Check sheet for the modelled part. Datum: model origin and axes. Units: mm. Face numbers are marked on the shaded views. A direction names the side the tool comes from. Coordinates: 2 decimals unless noted, no trailing zeros. Write each loop counter-clockwise with the first axis right and the second up, starting at its lowest first coordinate (ties: lowest second). Pieces come first, ordered by that corner, then holes. Notation, with made-up numbers: (77.25, 5) -> (127.25, 5) arc R21 cw to (127.25, 24) -> close; hole circle Ø5 at (10, 52.5). An arc over 180 degrees is marked (long way). One line per item, written item: value. Start each with the question number.
1) Sectioned sample at B-B on z = -14.25. Enter the section's corners in (x, y).
2) Sectioned sample at C-C on y = -8.25. Enter the section's corners in (x, z) (3 decimals), plus the area to 3 significant figures.
3) Sectioned sample at D-D on x = 11. Enter the section's corners in (y, z).
4) Set-up check for the marked faces 4, 5, 6, 7 and 8: record each of +Z, -Z, +X, -X, +Y, -Y from which the full face is reachable in a straight line by a thin tool's end or side.
5) Sectioned sample at A-A on x = 28. Enter the section's corners in (y, z).
6) Scan lines: line 1 along Y through (x, z) = (6, -6); line 2 along Z through (x, y) = (20, -3); line 3 along X through (y, z) = (-11.5, -10.75). Record each from-to range of solid material in increasing order. Write a range as [from, to].
7) Gauge pin test, flat ends, axial feed: P1, Ø4, axis at x = 27, y = -6, coming from the -Z side; P2, Ø11, axis at x = 25, z = 4, coming from the -Y side; P3, Ø1, axis at y = -15, z = 2, coming from the +X side; P4, Ø7.5, axis at x = -21.09, z = 1.52, coming from the +Y side. Record the tip position at first contact, or that the pin passes through.
8) Draft check along X on the marked faces 1, 2 and 3. Enter one of: +X half, -X half, draft (parallel to the pull), parting line (faces both ways), or undercut.
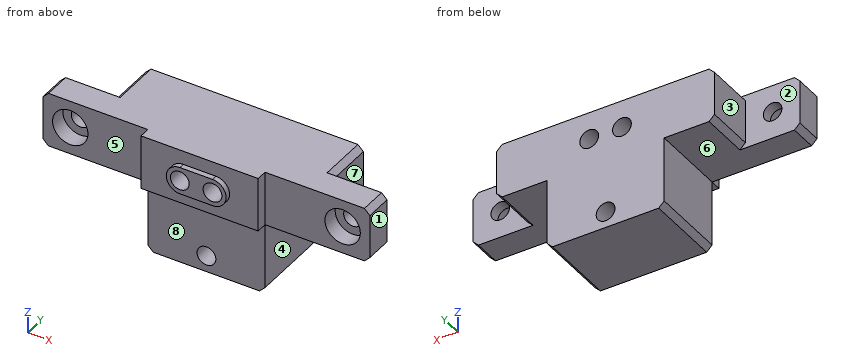
```python
from build123d import *

# Parameters (mm, degrees)
F1_DEPTH  = 16
F2_W      = 21.5
F2_H      = 13
F2_W_2    = 19.25
F2_H_2    = 10
F3_DEPTH  = 2
F4_R      = 3.25
F5_DEPTH  = 3
F6_R      = 1.7
F7_R      = 1.7
F8_DEPTH  = 25
F9_W      = 10
F9_H      = 10
F9_R      = 1.7
F10_DEPTH = 9
F13_DEPTH = 17
F11_R     = 1.725
F14_DEPTH = 15
F15_R     = 1.725
F16_DEPTH = 25
F17_SIZE  = 1


with BuildPart() as f1:
    # F0 (on Front) → F1 (new body)
    with BuildSketch(Plane.XZ):
        Polygon((33.9145704359, 6.5189368035), (-26.0854295641, 6.5189368035), (-26.0854295641, -3.4810631965), (-6.8354295641, -3.4810631965), (-6.8354295641, -16.4810631965), (14.6645704359, -16.4810631965), (14.6645704359, -3.4810631965), (33.9145704359, -3.4810631965), align=None)
    extrude(amount=F1_DEPTH)

    # F2 (on face) → F3 (cut)
    with BuildSketch(Plane.XZ.offset(16)):
        with Locations((3.9145704359, -9.9810631965)):
            Rectangle(F2_W, F2_H)
        with Locations((-16.4604295641, 1.5189368035)):
            Rectangle(F2_W_2, F2_H_2)
        with Locations((24.2895704359, 1.5189368035)):
            Rectangle(F2_W_2, F2_H_2)
    extrude(amount=-F3_DEPTH, mode=Mode.SUBTRACT)

    # F4 (on face) → F5 (cut)
    with BuildSketch(Plane.XZ.offset(14)):
        with Locations((-21.0854295641, 1.5189368035)):
            Circle(F4_R)
        with Locations((28.9145704359, 1.5189368035)):
            Circle(F4_R)
    extrude(amount=-F5_DEPTH, mode=Mode.SUBTRACT)

    # F6 (on face) + F7 (on face) → F8 (cut)
    with BuildSketch(Plane.XZ.offset(11)):
        with Locations((-21.0854295641, 1.5189368035)):
            Circle(F6_R)
    with BuildSketch(Plane.XZ.offset(11)):
        with Locations((28.9145704359, 1.5189368035)):
            Circle(F7_R)
    extrude(amount=-F8_DEPTH, mode=Mode.SUBTRACT)

    # F9 (on face) → F10 (cut)
    with BuildSketch(Plane(origin=(0, 0, 0), x_dir=(-1, 0, 0), z_dir=(0, 1, 0))):
        with Locations((21.0854295641, 1.5189368035)):
            Rectangle(F9_W, F9_H)
        with Locations((21.0854295641, 1.5189368035)):
            Circle(F9_R, mode=Mode.SUBTRACT)
        with Locations((-28.9145704359, 1.5189368035)):
            Rectangle(F9_W, F9_H)
        with Locations((-28.9145704359, 1.5189368035)):
            Circle(F9_R, mode=Mode.SUBTRACT)
    extrude(amount=-F10_DEPTH, mode=Mode.SUBTRACT)

    # F12 (on Front) → F13 (join)
    with BuildSketch(Plane.XZ):
        with BuildLine():
            Line((0.9346461738, -0.9810631965), (6.9134989753, -0.9810631965))
            ThreePointArc((6.9134989753, -0.9810631965), (9.4134989753, 1.5189368035), (6.9134989753, 4.0189368035))
            Line((6.9134989753, 4.0189368035), (0.9346461738, 4.0189368035))
            ThreePointArc((0.9346461738, 4.0189368035), (-1.5653538262, 1.5189368035), (0.9346461738, -0.9810631965))
        make_face()
    extrude(amount=F13_DEPTH)

    # F11 (on face) → F14 (cut, symmetric)
    with BuildSketch(Plane.XZ.offset(14)):
        with Locations((0.9145704359, 1.5189368035)):
            Circle(F11_R)
        with Locations((6.9145704359, 1.5189368035)):
            Circle(F11_R)
    extrude(amount=F14_DEPTH, both=True, mode=Mode.SUBTRACT)

    # F15 (on face) → F16 (cut)
    with BuildSketch(Plane.XZ.offset(14)):
        with Locations((3.9145704359, -13.4810631965)):
            Circle(F15_R)
    extrude(amount=-F16_DEPTH, mode=Mode.SUBTRACT)

    # F17
    f17_edges = [f1.edges().sort_by_distance(p)[0] for p in [
        (-6.83543, -7, -16.481063),
        (14.66457, -7, -16.481063),
        (33.91457, -11.5, -3.481063),
        (33.91457, -11.5, 6.518937),
        (-26.08543, -11.5, 6.518937),
        (-26.08543, -11.5, -3.481063),
        (-16.08543, -4.5, -3.481063),
        (-16.08543, -4.5, 6.518937),
        (23.91457, -4.5, 6.518937),
        (23.91457, -4.5, -3.481063),
    ]]
    chamfer(f17_edges, length=F17_SIZE)


solid = f1.part
```
Answers:
1. outline: (-6.84, -14) -> (2.37, -14) -> (2.37, 0) -> (-6.84, 0) -> close; (5.46, -14) -> (14.66, -14) -> (14.66, 0) -> (5.46, 0) -> close
2. outline: (-16.085, -2.481) -> (-15.085, -3.481) -> (-6.835, -3.481) -> (-6.835, -15.481) -> (-5.835, -16.481) -> (13.665, -16.481) -> (14.665, -15.481) -> (14.665, -3.481) -> (22.915, -3.481) -> (23.915, -2.481) -> (23.915, 5.519) -> (22.915, 6.519) -> (-15.085, 6.519) -> (-16.085, 5.519) -> close; hole circle Ø3.45 at (0.915, 1.519); hole circle Ø3.45 at (3.915, -13.481); hole circle Ø3.45 at (6.915, 1.519)
2. area: 648 mm2
3. outline: (-16, -3.48) -> (-14, -3.48) -> (-14, -16.48) -> (0, -16.48) -> (0, 6.52) -> (-16, 6.52) -> close
4. face 4: -Z, +X, +Y, -Y
4. face 5: +Z, -Z, -X, -Y
4. face 6: -Z, -X, +Y, -Y
4. face 7: +Z, -Z, +X, +Y
4. face 8: -Z, +X, -X, -Y
5. outline: (-14, -3.48) -> (-9, -3.48) -> (-9, 0.09) -> (-11, 0.09) -> (-11, -1.6) -> (-14, -1.6) -> close; (-14, 4.64) -> (-11, 4.64) -> (-11, 2.95) -> (-9, 2.95) -> (-9, 6.52) -> (-14, 6.52) -> close
6. line 1: y = [-14, 0]
6. line 2: z = [-3.48, 6.52]
6. line 3: x = [-6.84, 14.66]
7. P1: passes through
7. P2: stops at y = -14
7. P3: stops at x = 14.66
7. P4: stops at y = -9
8. face 1: +X half
8. face 2: draft
8. face 3: -X half
